Verification items for this drawing (mm, ordinates from the low corner). Round coordinates to 2 decimals unless told otherwise and drop trailing zeros. Loops run counter-clockwise (first coordinate to the right, second up) from the corner with the lowest first, then second, coordinate; pieces in that order, holes last. Notation, with made-up numbers: (60, 0.5) -> (86, 0.5) arc R26 ccw to (86, 25.5) -> close; hole circle Ø2 at (41, -7). An arc over 180 degrees is marked (long way). One line per question, with ' | ' between items.
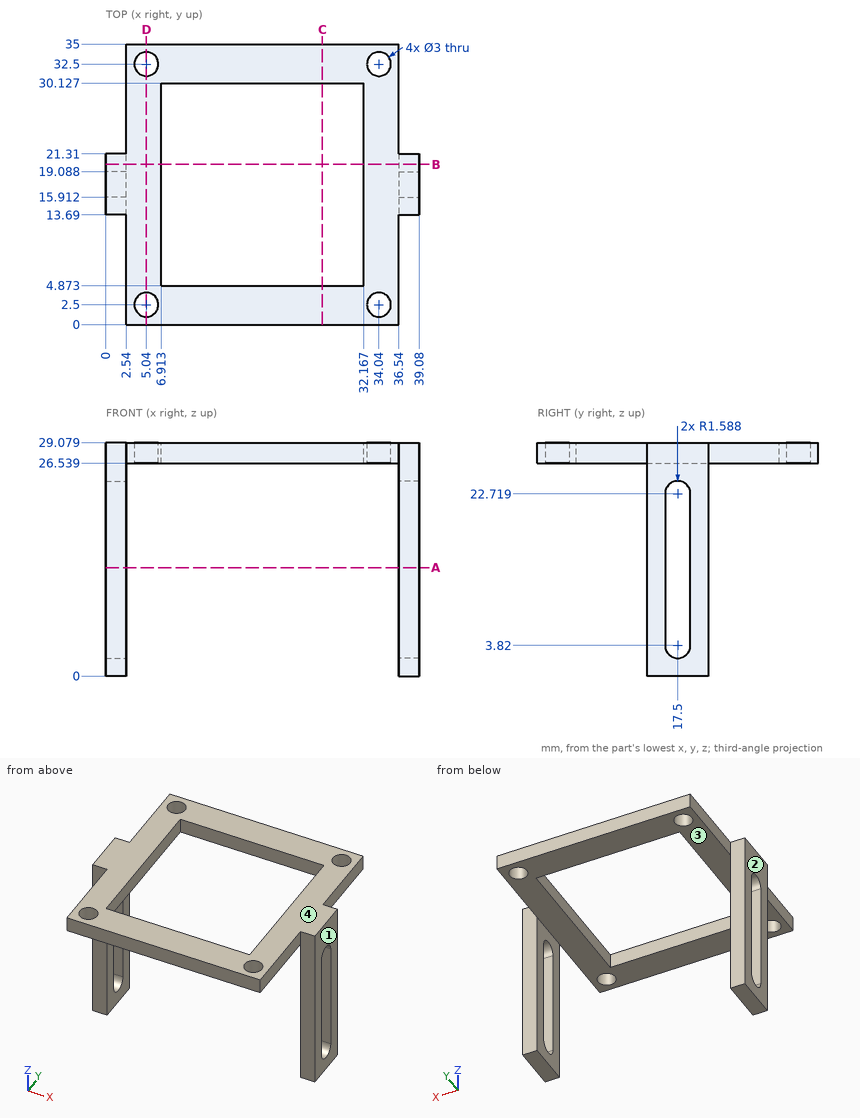
(1) Sectioned sample at D-D, the plane x = 5.04. Record the cut outline in (y, z).
Answer:
outline: (0, 26.54) -> (1, 26.54) -> (1, 29.08) -> (0, 29.08) -> close; (4, 26.54) -> (31, 26.54) -> (31, 29.08) -> (4, 29.08) -> close; (34, 26.54) -> (35, 26.54) -> (35, 29.08) -> (34, 29.08) -> close
(2) Scan lines: probe 1 along Y at (x, z) = (34.04, 27.55); probe 2 along X at (y, z) = (19.5, 4.5); probe 3 along Z at (x, y) = (13, 2). Record each from-to range of solid material in increasing order.
Answer:
probe 1: y = 0 to 1, 4 to 31, 34 to 35 | probe 2: x = 0 to 2.54, 36.54 to 39.08 | probe 3: z = 26.54 to 29.08
(3) Sectioned sample at A-A, the plane z = 13.5. Record the cut outline in (x, y).
Answer:
outline: (0, 13.69) -> (2.54, 13.69) -> (2.54, 15.91) -> (0, 15.91) -> close; (0, 19.09) -> (2.54, 19.09) -> (2.54, 21.31) -> (0, 21.31) -> close; (36.54, 13.69) -> (39.08, 13.69) -> (39.08, 15.91) -> (36.54, 15.91) -> close; (36.54, 19.09) -> (39.08, 19.09) -> (39.08, 21.31) -> (36.54, 21.31) -> close
(4) Go/stop test with flat-tipped pins: pin 1 (3 mm diameter, centred on y = 6, z = 28.5, fed in from -X); pin 2 (0.8 mm diameter, centred on y = 22, z = 28, fed in from +X); pin 3 (3 mm diameter, centred on x = 37, z = 14, fed in from -Y); pin 4 (2.5 mm diameter, centred on y = 16, z = 8, fed in from +X). Record where each tip stops, or that it passes through.
Answer:
pin 1: stops at x = 2.54 | pin 2: stops at x = 36.54 | pin 3: stops at y = 13.69 | pin 4: stops at x = 39.08
(5) Sectioned sample at C-C, the plane x = 27. Record the cut outline in (y, z).
Answer:
outline: (0, 26.54) -> (4.87, 26.54) -> (4.87, 29.08) -> (0, 29.08) -> close; (30.13, 26.54) -> (35, 26.54) -> (35, 29.08) -> (30.13, 29.08) -> close
(6) Mould release check, pull along X, two halves, no side actions. Record for the marked faces 1, 2, 3 and 4: +X half, -X half, draft (parallel to the pull), parting line (faces both ways), or undercut.
Answer:
face 1: +X half | face 2: -X half | face 3: undercut | face 4: draft
(7) Sectioned sample at B-B, the plane y = 20. Record the cut outline in (x, z), and give its area (3 significant figures).
Answer:
outline: (0, 0) -> (2.54, 0) -> (2.54, 26.54) -> (6.91, 26.54) -> (6.91, 29.08) -> (0, 29.08) -> close; (32.17, 26.54) -> (36.54, 26.54) -> (36.54, 0) -> (39.08, 0) -> (39.08, 29.08) -> (32.17, 29.08) -> close | area: 170 mm2
